Read the model definition and answer for the solid it produces. Units are mm, in the model's axes. Face numbers are marked on the shaded views. A direction names the side the tool comes from. Give positions to 0.01 mm unless a question says otherwise; leave off trailing zeros. Order: outer loops, then holes, each group sorted by start corner. A loop starts at its lowest first (then second) coordinate and runs counter-clockwise, first axis right, second up. Notation, with made-up numbers: (46.5, -38) - (78.5, -38) arc R20 cw to (78.5, -7) - close; hole circle Ø4 at (64, 70.5). An arc over 180 degrees is marked (long way). Use a Markdown table: item, result. Add a question column.
1. Consider L1, parallel to Z at x = 1, y = -1; L2, parallel to X at y = 16.5, z = -21.5; L3, parallel to X at y = -40.5, z = 11. Determine where each line is inside the solid, lowest interval first.
2. A cutting plane is placed at A-A on z = 0. State how many separate pieces and enclosed holes the cut face has, and give its area (3 significant figures).
3. A cutting plane is placed at C-C on x = 6.5. Determine the outline of the cut face in (y, z), and give its area (3 significant figures).
4. Which of the six approach directions +Z, -Z, +X, -X, +Y, -Y give full straight-line access (tool end or side, diameter ignored) to the marked faces 1 and 2?
5. Flat-ended cylindrical pins translate along their axes: P1, Ø7, axis at y = -28.28, z = 28.28, coming from the -X side; P2, Ø5, axis at x = 9.5, z = -10.5, coming from the +Y side; P3, Ø3, axis at x = 2.5, y = -6, coming from the +Z side; P4, Ø12, axis at y = -6, z = 24, coming from the -X side. Find the tip coordinate at first contact, or state that the pin passes through.
6. For a pull along Y with two mould halves and no side action, classify the marked faces 3 and 4 as released by +Y, released by -Y, zero draft, split by the parting line, or undercut.
```python
from build123d import *

# Parameters (mm, degrees)
SKETCH_3_R          = 3
CUT_EXTRUDE_1_DEPTH = 10
CHAMFER_1_SIZE      = 0.5
FILLET_1_R          = 5


with BuildPart() as part:
    # 草图1 → 旋转1 (revolve)
    with BuildSketch(Plane.XY):
        Polygon((0, 0), (0, 30), (8, 30), (8, 45), (14, 45), (14, 27.5), (16, 27.5), (16, 0), align=None)
    revolve(axis=Axis((16, 0, 0), (-1, 0, 0)))

    # 草图2 → 切除-旋转1 (revolve, cut)
    with BuildSketch(Plane.XY, mode=Mode.PRIVATE) as cut_revolve_1_sk:
        Polygon((0, 0), (0, 27.5), (10, 27.5), (10, 24), (16, 24), (16, 0), align=None)
    revolve(cut_revolve_1_sk.sketch.rotate(Axis((16, 0, 0), (-1, 0, 0)), 90), axis=Axis((16, 0, 0), (-1, 0, 0)), mode=Mode.SUBTRACT)

    # 草图3 → 切除-拉伸1 (cut)
    with BuildSketch(Plane.ZY.offset(-8)):
        with Locations(Location((0, 40, 0), (0, 0, 270))):
            Circle(SKETCH_3_R)
        with Locations(Location((28.284271247, 28.284271247, 0), (0, 0, 270))):
            Circle(SKETCH_3_R)
        with Locations(Location((40, 0, 0), (0, 0, 270))):
            Circle(SKETCH_3_R)
        with Locations(Location((28.284271247, -28.284271247, 0), (0, 0, 270))):
            Circle(SKETCH_3_R)
        with Locations(Location((0, -40, 0), (0, 0, 270))):
            Circle(SKETCH_3_R)
        with Locations(Location((-28.284271247, -28.284271247, 0), (0, 0, 270))):
            Circle(SKETCH_3_R)
        with Locations(Location((-40, 0, 0), (0, 0, 270))):
            Circle(SKETCH_3_R)
        with Locations(Location((-28.284271247, 28.284271247, 0), (0, 0, 270))):
            Circle(SKETCH_3_R)
    extrude(amount=-CUT_EXTRUDE_1_DEPTH, mode=Mode.SUBTRACT)

    # 倒角1
    chamfer_1_edges = [part.edges().sort_by_distance(p)[0] for p in [
        (14, -45, 0),
        (8, -45, 0),
        (0, -30, 0),
    ]]
    chamfer(chamfer_1_edges, length=CHAMFER_1_SIZE)

    # 圆角1
    fillet_1_edges = [part.edges().sort_by_distance(p)[0] for p in [
        (8, -30, 0),
    ]]
    fillet(fillet_1_edges, radius=FILLET_1_R)


solid = part.part
```
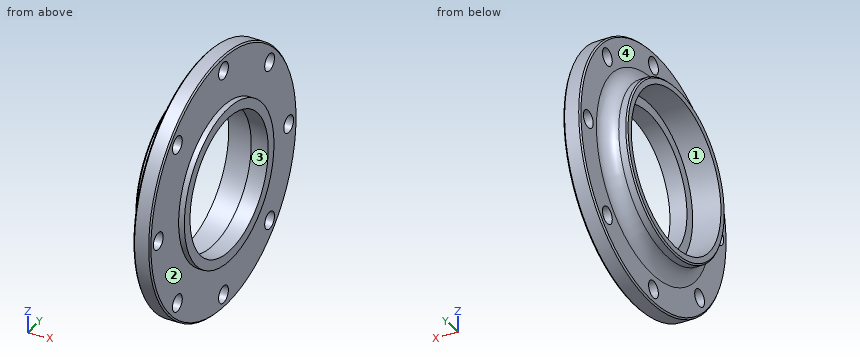
Output values:
| question | item | result |
|---|---|---|
| 1 | L1 | -29.98 to -27.48, 27.48 to 29.98 |
| 1 | L2 | 10 to 16 |
| 1 | L3 | 8 to 14 |
| 2 | separate pieces | 4 |
| 2 | enclosed holes | 0 |
| 2 | area | 230 mm² |
| 3 | outline | circle Ø62.86 at (0, 0); hole circle Ø55 at (0, 0) |
| 3 | area | 727 mm² |
| 4 | face 1 | -X |
| 4 | face 2 | +X |
| 5 | P1 | x = 8 |
| 5 | P2 | y = 44.28 |
| 5 | P3 | z = 29.66 |
| 5 | P4 | x = 0 |
| 6 | face 3 | undercut |
| 6 | face 4 | zero draft |
